from build123d import *

# Parameters (mm, degrees)
ESQUISSE1_W              = 52
ESQUISSE1_H              = 50
BOSS_EXTRU_1_DEPTH       = 2
EMPREINTE1_START         = -50
EMPREINTE1_OUTLINE_W     = 2.02
EMPREINTE1_OUTLINE_H     = 2
EMPREINTE1_OUTLINE_W_2   = 49.9598
EMPREINTE1_DEPTH         = 2.02
EMPREINTE1_START_2       = -2
EMPREINTE1_2_OUTLINE_W   = 2.02
EMPREINTE1_2_OUTLINE_H   = 2
EMPREINTE1_2_OUTLINE_W_2 = 49.9598
EMPREINTE1_2_DEPTH       = 2
EMPREINTE1_START_3       = -17.67235879
EMPREINTE1_3_OUTLINE_W   = 2.02
EMPREINTE1_3_OUTLINE_H   = 2
EMPREINTE1_3_OUTLINE_W_2 = 2
EMPREINTE1_3_DEPTH       = 15.67235879
EMPREINTE1_START_4       = -47.98
EMPREINTE1_4_OUTLINE_W   = 2.02
EMPREINTE1_4_OUTLINE_H   = 2
EMPREINTE1_4_OUTLINE_W_2 = 2
EMPREINTE1_4_DEPTH       = 15.15235879
ESQUISSE2_W              = 9.61940452
ESQUISSE2_H              = 3.700848348
ESQUISSE2_W_2            = 14.786584651
ESQUISSE2_H_2            = 4.070824207
ENL_V_MAT_EXTRU_1_DEPTH  = 2


# Read off the part's stored shape, not the designer's step: Empreinte1
with BuildPart() as part:
    # Esquisse1 → Boss.-Extru.1 (new body)
    with BuildSketch(Plane(origin=(0, 0, 0), x_dir=(1, 0, 0), z_dir=(0, 1, 0))):
        with Locations((26, 25)):
            Rectangle(ESQUISSE1_W, ESQUISSE1_H)
    extrude(amount=BOSS_EXTRU_1_DEPTH)

    # Empreinte1 outline → Empreinte1 (cut)
    with BuildSketch(Plane.XY.offset(EMPREINTE1_START)):
        with Locations((1.01, 1)):
            Rectangle(EMPREINTE1_OUTLINE_W, EMPREINTE1_OUTLINE_H)
        with Locations((27.0201, 1)):
            Rectangle(EMPREINTE1_OUTLINE_W_2, EMPREINTE1_OUTLINE_H)
    extrude(amount=EMPREINTE1_DEPTH, mode=Mode.SUBTRACT)

    # Empreinte1 2 outline → Empreinte1 2 (cut)
    with BuildSketch(Plane.XY.offset(EMPREINTE1_START_2)):
        with Locations((1.01, 1)):
            Rectangle(EMPREINTE1_2_OUTLINE_W, EMPREINTE1_2_OUTLINE_H)
        with Locations((27.0201, 1)):
            Rectangle(EMPREINTE1_2_OUTLINE_W_2, EMPREINTE1_2_OUTLINE_H)
    extrude(amount=EMPREINTE1_2_DEPTH, mode=Mode.SUBTRACT)

    # Empreinte1 3 outline → Empreinte1 3 (cut)
    with BuildSketch(Plane.XY.offset(EMPREINTE1_START_3)):
        with Locations((1.01, 1)):
            Rectangle(EMPREINTE1_3_OUTLINE_W, EMPREINTE1_3_OUTLINE_H)
        with Locations((51, 1)):
            Rectangle(EMPREINTE1_3_OUTLINE_W_2, EMPREINTE1_3_OUTLINE_H)
    extrude(amount=EMPREINTE1_3_DEPTH, mode=Mode.SUBTRACT)

    # Empreinte1 4 outline → Empreinte1 4 (cut)
    with BuildSketch(Plane.XY.offset(EMPREINTE1_START_4)):
        with Locations((1.01, 1)):
            Rectangle(EMPREINTE1_4_OUTLINE_W, EMPREINTE1_4_OUTLINE_H)
        with Locations((51, 1)):
            Rectangle(EMPREINTE1_4_OUTLINE_W_2, EMPREINTE1_4_OUTLINE_H)
    extrude(amount=EMPREINTE1_4_DEPTH, mode=Mode.SUBTRACT)

    # Esquisse2 → Enlèv. mat.-Extru.1 (cut)
    with BuildSketch(Plane(origin=(0, 2, 0), x_dir=(1, 0, 0), z_dir=(0, 1, 0))):
        with Locations((1.626508817, 49.830424174)):
            Rectangle(ESQUISSE2_W, ESQUISSE2_H)
        with Locations((5.120042554, -0.035412104)):
            Rectangle(ESQUISSE2_W_2, ESQUISSE2_H_2)
    extrude(amount=-ENL_V_MAT_EXTRU_1_DEPTH, mode=Mode.SUBTRACT)


solid = part.part
The model under review builds one solid part; all positions refer to its coordinate system, in mm. A direction names the side the tool comes from. Give positions to 0.01 mm unless a question says otherwise; leave off trailing zeros. Write each loop counter-clockwise with the first axis right and the second up, starting at its lowest first coordinate (ties: lowest second). Pieces come first, ordered by that corner, then holes.
1. Wall thickness on L1, parallel to X at y = 0.6, z = -39: over which ranges is the line inside the solid? List them lowest first.
2. Add section A-A, the plane y = 0.85. Write out the cut boundary in (x, z), plus the area to 3 significant figures.
3. For P1, Ø1, axis at y = 1, z = -37.5, coming from the -X side, flat-tipped, find the tip position at first contact; note if it passes through.
4. Tool access review of faces 1 (the flat face through (2.02, 1, -41)), 2 (the flat face through (51, 1, -32.828)), 3 (the flat face through (51, 1, -17.672)), 4 (the flat face through (1, 1, -17.672)), 5 (the flat face through (26, 1, -2)): name each direction out of +Z, -Z, +X, -X, +Y, -Y from which nothing blocks a thin tool from reaching the whole face with its end or side.
5. Add section B-B, the plane z = -13.5. Write out the cut boundary in (x, y).
Worked answers:
1. L1: x = 2.02 to 50
2. outline: (0, -32.83) - (2.02, -32.83) - (2.02, -47.98) - (50, -47.98) - (50, -32.83) - (52, -32.83) - (52, -17.67) - (50, -17.67) - (50, -2) - (2.02, -2) - (2.02, -17.67) - (0, -17.67) - close
2. area: 2,270 mm2
3. P1: stops at x = 2.02
4. face 1: -Z, -X, +Y, -Y
4. face 2: -Z, +X, +Y, -Y
4. face 3: +Z, +X, +Y, -Y
4. face 4: +Z, -X, +Y, -Y
4. face 5: +Z, +X, -X, +Y, -Y
5. outline: (2.02, 0) - (50, 0) - (50, 2) - (2.02, 2) - close
